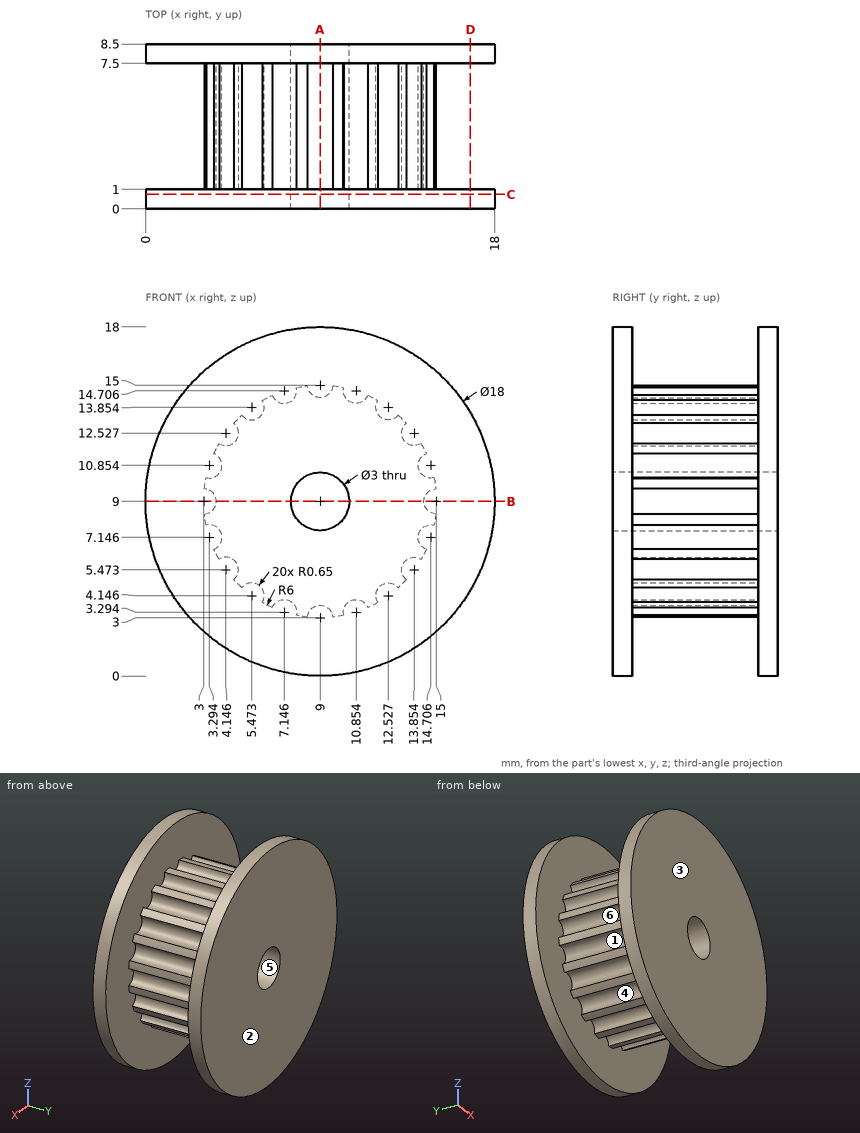
Verification items for this drawing (mm, ordinates from the low corner). A direction names the side the tool comes from. Round coordinates to 2 decimals unless told otherwise and drop trailing zeros. Loops run counter-clockwise (first coordinate to the right, second up) from the corner with the lowest first, then second, coordinate; pieces in that order, holes last. Notation, with made-up numbers: (71, 71) - (126, 71) arc R20 ccw to (126, 78) - close; hole circle Ø6 at (78.5, -36). An arc over 180 degrees is marked (long way). Answer as CSV lines item,"result". Start each with the question number.
Item 1: Depth check by flat-ended pin: P1, Ø2, axis at x = 10, z = 8.5, coming from the +Y side; P2, Ø4, axis at y = 2, z = 12.5, coming from the +X side (1 decimal); P3, Ø4, axis at y = 4, z = 9, coming from the +X side (1 decimal); P4, Ø5, axis at x = 2.5, y = 1, coming from the -Z side. Enter the tip coordinate at first touch or a pass-through.
Item 2: Release check for a two-part mould opening along Y. For the marked faces 1, 2 and 3 record: +Y half, -Y half, draft (parallel to the pull), parting line (faces both ways), or undercut.
Item 3: Scan lines: line 1 (Y direction, x = 9, z = 17); line 2 (X direction, y = 4.5, z = 9); line 3 (Z direction, x = 9.5, y = 2) (1 decimal). Record each from-to range of solid material in increasing order. Write a range as [from, to].
Item 4: Section check D-D (x = 16.75). Record the boundary of the cut face in (y, z).
Item 5: Section check B-B (z = 9). Record the boundary of the cut face in (x, y).
Item 6: Section check A-A (x = 9). Record the boundary of the cut face in (y, z).
Item 7: Section check C-C (y = 0.75). Record the boundary of the cut face in (x, z).
Item 8: Set-up check for the marked faces 4, 5 and 6: record each of +Z, -Z, +X, -X, +Y, -Y from which the full face is reachable in a straight line by a thin tool's end or side.
Report:
1,P1,"stops at y = 8.5"
1,P2,"stops at x = 17.8"
1,P3,"stops at x = 15"
1,P4,"stops at z = 0.94"
2,face 1,"undercut"
2,face 2,"+Y half"
2,face 3,"-Y half"
3,line 1,"y = [0, 1], [7.5, 8.5]"
3,line 2,"x = [3.65, 7.5], [10.5, 14.35]"
3,line 3,"z = [3.4, 7.6], [10.4, 14.6]"
4,outline,"(0, 4.42) - (1, 4.42) - (1, 13.58) - (0, 13.58) - close; (7.5, 4.42) - (8.5, 4.42) - (8.5, 13.58) - (7.5, 13.58) - close"
5,outline,"(0, 0) - (7.5, 0) - (7.5, 8.5) - (0, 8.5) - (0, 7.5) - (3.65, 7.5) - (3.65, 1) - (0, 1) - close; (10.5, 0) - (18, 0) - (18, 1) - (14.35, 1) - (14.35, 7.5) - (18, 7.5) - (18, 8.5) - (10.5, 8.5) - close"
6,outline,"(0, 0) - (1, 0) - (1, 3.65) - (7.5, 3.65) - (7.5, 0) - (8.5, 0) - (8.5, 7.5) - (0, 7.5) - close; (0, 10.5) - (8.5, 10.5) - (8.5, 18) - (7.5, 18) - (7.5, 14.35) - (1, 14.35) - (1, 18) - (0, 18) - close"
7,outline,"circle Ø18 at (9, 9); hole circle Ø3 at (9, 9)"
8,face 4,"none"
8,face 5,"+Y, -Y"
8,face 6,"-X"
